Can you work these out from the model? Positions are in its coordinate system, mm. A direction names the side the tool comes from. Give positions to 0.01 mm unless a question says otherwise; leave off trailing zeros. Loops run counter-clockwise (first coordinate to the right, second up) from the corner with the lowest first, then second, coordinate; pieces in that order, holes last.
from build123d import *

# Parameters (mm, degrees)
SKETCH1_R           = 2.5
BOSS_EXTRUDE2_DEPTH = 4
SKETCH14_W          = 10
SKETCH14_H          = 4
BOSS_EXTRUDE5_DEPTH = 4
SKETCH15_W          = 10
SKETCH15_H          = 4
BOSS_EXTRUDE6_DEPTH = 4


with BuildPart() as part:
    # Sketch1 → Boss-Extrude2 (new body)
    with BuildSketch(Plane(origin=(0, 0, 0), x_dir=(1, 0, 0), z_dir=(0, 1, 0))):
        Polygon((36.786877756, 11.613831083), (44.492502068, 11.613831083), (44.492502068, -11.613831083), (36.786877756, -11.613831083), (27.518556454, -11.613831083), (12.70818574, -11.613831083), (12.70818574, 11.613831083), (27.518556454, 11.613831083), align=None)
        with Locations((16.5, 0)):
            Circle(SKETCH1_R, mode=Mode.SUBTRACT)
        with Locations((22.5, 0)):
            Circle(SKETCH1_R, mode=Mode.SUBTRACT)
        with Locations((28.5, 0)):
            Circle(SKETCH1_R, mode=Mode.SUBTRACT)
        with Locations((34.5, 0)):
            Circle(SKETCH1_R, mode=Mode.SUBTRACT)
    extrude(amount=BOSS_EXTRUDE2_DEPTH)

    # Sketch14 → Boss-Extrude5 (add)
    with BuildSketch(Plane.XY.offset(11.613831083)):
        with Locations((28.600343904, 2)):
            Rectangle(SKETCH14_W, SKETCH14_H)
    extrude(amount=BOSS_EXTRUDE5_DEPTH)

    # Sketch15 → Boss-Extrude6 (add)
    with BuildSketch(Plane(origin=(0, 0, -11.613831083), x_dir=(-1, 0, 0), z_dir=(0, 0, -1))):
        with Locations((-28.600343904, 2)):
            Rectangle(SKETCH15_W, SKETCH15_H)
    extrude(amount=BOSS_EXTRUDE6_DEPTH)


solid = part.part
(1) Suppose I cut it at C-C on y = 1.45. List the corners of the cut face in (x, z) for me.
Returned:
outline: (12.71, -11.61) - (23.6, -11.61) - (23.6, -15.61) - (33.6, -15.61) - (33.6, -11.61) - (44.49, -11.61) - (44.49, 11.61) - (33.6, 11.61) - (33.6, 15.61) - (23.6, 15.61) - (23.6, 11.61) - (12.71, 11.61) - close; hole circle Ø5 at (16.5, 0); hole circle Ø5 at (22.5, 0); hole circle Ø5 at (28.5, 0); hole circle Ø5 at (34.5, 0)
(2) Which directions (+Z, -Z, +X, -X, +Y, -Y) give clear straight access to the entire face, cutting with the end or side of a thin tool? Please do faces 1 (the flat face through (18, 2, 11.614)), 2 (the flat face through (29, 4, -4)), 3 (the flat face through (23.6, 2, -14)), 4 (the flat face through (39, 2, -11.614)), 5 (the flat face through (33.6, 2, 14)).
Returned:
face 1: +Z, -X, +Y, -Y
face 2: +Z, -Z, +X, -X, +Y
face 3: -Z, -X, +Y, -Y
face 4: -Z, +X, +Y, -Y
face 5: +Z, +X, +Y, -Y
(3) Suppose I cut it at A-A on z = -2. List the corners of the cut face in (x, y) for me.
Returned:
outline: (12.71, 0) - (15, 0) - (15, 4) - (12.71, 4) - close; (18, 0) - (21, 0) - (21, 4) - (18, 4) - close; (24, 0) - (27, 0) - (27, 4) - (24, 4) - close; (30, 0) - (33, 0) - (33, 4) - (30, 4) - close; (36, 0) - (44.49, 0) - (44.49, 4) - (36, 4) - close
(4) Please list where these lines run through material, in increasing order: probe 1 along X at (y, z) = (1.55, 0); probe 2 along Z at (x, y) = (28.5, 2.6); probe 3 along Z at (x, y) = (34.5, 0.85).
Returned:
probe 1: x = 12.71 to 14, 19 to 20, 25 to 26, 31 to 32, 37 to 44.49
probe 2: z = -15.61 to -2.5, 2.5 to 15.61
probe 3: z = -11.61 to -2.5, 2.5 to 11.61
(5) Suppose I cut it at B-B on x = 28.5. List the corners of the cut face in (y, z) for me.
Returned:
outline: (0, -15.61) - (4, -15.61) - (4, -2.5) - (0, -2.5) - close; (0, 2.5) - (4, 2.5) - (4, 15.61) - (0, 15.61) - close
(6) Suppose I cut it at D-D on x = 34.5. List the corners of the cut face in (y, z) for me.
Returned:
outline: (0, -11.61) - (4, -11.61) - (4, -2.5) - (0, -2.5) - close; (0, 2.5) - (4, 2.5) - (4, 11.61) - (0, 11.61) - close
(7) Will these pins go through, and if not, where does the flat tip stop? P1, Ø2, axis at y = 3, z = -14.5, coming from the +X side; P2, Ø1.2, axis at x = 20, y = 1, coming from the +Z side; P3, Ø2, axis at x = 39, y = 2, coming from the -Z side; P4, Ø3, axis at x = 28.5, z = 0, coming from the -Y side.
Returned:
P1: stops at x = 33.6
P2: stops at z = 11.61
P3: stops at z = -11.61
P4: passes through
(8) Thinking about a two-plate mould opening in X: for faces 6 (the flat face through (23.6, 2, 14)), 7 (the cylindrical face through (20, 2, 0)), 8 (the flat face through (29, 2, 15.614)), which applies, pulls with the +X half, pulls with the -X half, needs draft (parallel to the pull), parting line crosses it, or undercut?
Returned:
face 6: pulls with the -X half
face 7: undercut
face 8: needs draft
